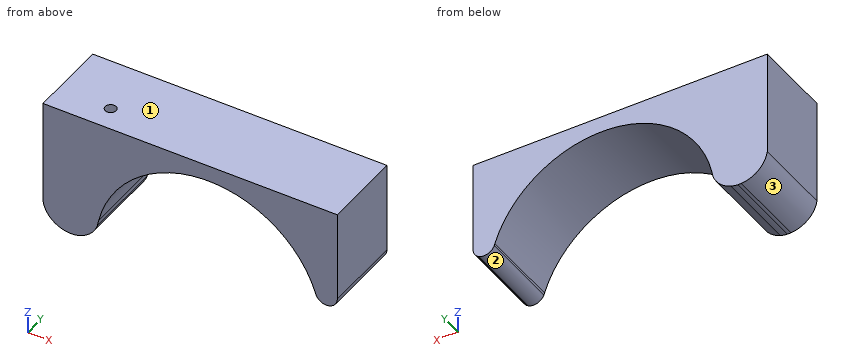
from build123d import *

# Parameters (mm, degrees)
F1_DEPTH = 15.875
F2_R     = 1.0922
F3_DEPTH = 12.7


# Not quite as in the source:
# - ends of sketch curves that miss each other by under 0.0002 mm in the source are joined


with BuildPart() as f1:
    # F0 (on Front) → F1 (new body)
    with BuildSketch(Plane.XZ):
        with BuildLine():
            ThreePointArc((21.0836389118, 7.0307037512), (21.1482213946, 6.8339854292), (21.2109684651, 6.6366739991))
            ThreePointArc((21.2109684651, 6.6366739991), (22.5210215532, 5.4318172042), (24.2927235367, 5.6020848515))
            Line((24.2927235367, 5.6020848515), (24.5564028335, 5.7779212439))
            ThreePointArc((24.5564028335, 5.7779212439), (24.6317726398, 5.83924537), (24.7043401509, 5.9038612541))
            ThreePointArc((24.7043401509, 5.9038612541), (24.1693958795, 7.8102690619), (23.4875772319, 9.6692148479))
            ThreePointArc((23.4875772319, 9.6692148479), (21.6017035502, 8.9730623402), (21.0836389118, 7.0307037512))
        make_face()
        with BuildLine():
            ThreePointArc((-25.3984668781, 0.2790703183), (-23.2092642977, 1.6544209311), (-21.8846396204, 3.8746836882))
            ThreePointArc((-21.8846396204, 3.8746836882), (-21.7800085202, 4.4251388519), (-21.6615343316, 4.9727814551))
            ThreePointArc((-21.6615343316, 4.9727814551), (-21.6412555699, 5.2455472098), (-21.6344904646, 5.5189820621))
            ThreePointArc((-21.6344904646, 5.5189820621), (-22.1206425964, 7.786095443), (-23.4936109358, 9.6545453128))
            ThreePointArc((-23.4936109358, 9.6545453128), (-24.8914383088, 5.057301545), (-25.3984668781, 0.2790703183))
        make_face()
        with BuildLine():
            Line((0, 25.4), (0, 22.225))
            ThreePointArc((0, 22.225), (12.9940993172, 18.0306408077), (21.0836389118, 7.0307037512))
            ThreePointArc((21.0836389118, 7.0307037512), (21.6017035502, 8.9730623402), (23.4875772319, 9.6692148479))
            ThreePointArc((23.4875772319, 9.6692148479), (14.1343896731, 21.1040050362), (0, 25.4))
        make_face()
        with BuildLine():
            ThreePointArc((-21.6615343316, 4.9727814551), (-13.8461286495, 17.3849172106), (0, 22.225))
            Line((0, 22.225), (0, 25.4))
            ThreePointArc((0, 25.4), (-14.1409785562, 21.099590647), (-23.4936109358, 9.6545453128))
            ThreePointArc((-23.4936109358, 9.6545453128), (-22.1206425964, 7.786095443), (-21.6344904646, 5.5189820621))
            ThreePointArc((-21.6344904646, 5.5189820621), (-21.6412555699, 5.2455472098), (-21.6615343316, 4.9727814551))
        make_face()
        with BuildLine():
            ThreePointArc((-26.8263954087, 0), (-26.1032119587, 0.0923630453), (-25.3984668781, 0.2790703183))
            ThreePointArc((-25.3984668781, 0.2790703183), (-24.8914383088, 5.057301545), (-23.4936109358, 9.6545453128))
            ThreePointArc((-23.4936109358, 9.6545453128), (-29.0403261825, 10.7200919312), (-32.6289507574, 6.3585310541))
            Line((-32.6289507574, 6.3585310541), (-32.6289507574, 4.6794330701))
            ThreePointArc((-32.6289507574, 4.6794330701), (-30.8909302127, 1.4347070449), (-27.501154691, 0))
            Line((-27.501154691, 0), (-26.8263954087, 0))
        make_face()
        with BuildLine():
            ThreePointArc((23.4875772319, 9.6692148479), (24.1693958795, 7.8102690619), (24.7043401509, 5.9038612541))
            ThreePointArc((24.7043401509, 5.9038612541), (25.2185681707, 6.630615454), (25.4000290489, 7.5022082908))
            ThreePointArc((25.4000290489, 7.5022082908), (24.8535428533, 8.9473198237), (23.4875772319, 9.6692148479))
        make_face()
        with BuildLine():
            ThreePointArc((23.4875772319, 9.6692148479), (24.8535428533, 8.9473198237), (25.4000290489, 7.5022082908))
            Line((25.4000290489, 7.5022082908), (25.4, 25.4))
            Line((25.4, 25.4), (0, 25.4))
            ThreePointArc((0, 25.4), (14.1343896731, 21.1040050362), (23.4875772319, 9.6692148479))
        make_face()
        with BuildLine():
            ThreePointArc((-23.4936109358, 9.6545453128), (-14.1409785562, 21.099590647), (0, 25.4))
            Line((0, 25.4), (-25.3993433231, 25.4))
            Line((-25.3993433231, 25.4), (-32.6289507574, 25.4))
            Line((-32.6289507574, 25.4), (-32.6289507574, 6.3585310541))
            ThreePointArc((-32.6289507574, 6.3585310541), (-29.0403261825, 10.7200919312), (-23.4936109358, 9.6545453128))
        make_face()
    extrude(amount=F1_DEPTH)

    # F2 (on face) → F3 (cut)
    with BuildSketch(Plane.XY.offset(25.4)):
        with Locations((-22.225, -11.1125)):
            Circle(F2_R)
    extrude(amount=-F3_DEPTH, mode=Mode.SUBTRACT)


solid = f1.part
Verification items for the finished model (mm, model axes). Face numbers are marked on the shaded views. Coordinates: 2 decimals unless noted, no trailing zeros. Write each loop counter-clockwise with the first axis right and the second up, starting at its lowest first coordinate (ties: lowest second). Pieces come first, ordered by that corner, then holes. Notation, with made-up numbers: M 16,-2 L 33,-2 A21 ccw 33,27 Z; hole C 66.5,26 d7. An arc over 180 degrees is marked long. Use CSV: the item, a comma, the result in double quotes.
Q1. Section check D-D, the plane x = 2. Enter the section's corners in (y, z) (3 decimals).
Computed values:
outline,"M -15.875,22.135 L 0,22.135 L 0,25.4 L -15.875,25.4 Z"
Q2. Thickness scan on line 1 along X through (y, z) = (-3.25, 7); line 2 along X through (y, z) = (-9.5, 7.25); line 3 along Z through (x, y) = (7, -1.5). Record the ranges inside material, lowest first. Write a range as [from, to].
Computed values:
line 1,"[-32.63, -21.09], [21.09, 25.34]"
line 2,"[-32.63, -21.01], [21.01, 25.39]"
line 3,"[21.09, 25.4]"
Q3. Go/stop test with flat-tipped pins: P1, Ø6, axis at x = 13, y = -2, coming from the -Z side; P2, Ø2.5, axis at x = -22.22, y = -11.11, coming from the -Z side; P3, Ø0.7, axis at x = -21.5, y = -11.5, coming from the +Z side; P4, Ø8, axis at x = -8.5, y = -13.5, coming from the -Z side. Record where each tip stops, or that it passes through.
Computed values:
P1,"z = 15.43"
P2,"z = 1.4"
P3,"z = 25.4"
P4,"z = 18.38"
Q4. Section check C-C, the plane z = 11.5. Enter the section's corners in (x, y) (3 decimals), and give its area (3 significant figures).
Computed values:
outline,"M -32.629,-15.875 L -19.018,-15.875 L -19.018,0 L -32.629,0 Z; M 19.018,-15.875 L 25.4,-15.875 L 25.4,0 L 19.018,0 Z"
area,"317 mm²"
Q5. Section check A-A, the plane z = 19. Enter the section's corners in (x, y) (1 decimal).
Computed values:
outline,"M -32.6,-15.9 L -11.5,-15.9 L -11.5,0 L -32.6,0 Z; M 11.5,-15.9 L 25.4,-15.9 L 25.4,0 L 11.5,0 Z; hole C -22.2,-11.1 d2.2"
Q6. Mould release check, pull along X, two halves, no side actions. Record for the marked faces 1, 2 and 3: pulls with the +X half, pulls with the -X half, needs draft (parallel to the pull), parting line crosses it, or undercut.
Computed values:
face 1,"needs draft"
face 2,"undercut"
face 3,"pulls with the -X half"
Q7. Section check B-B, the plane y = -5. Enter the section's corners in (x, z) (3 decimals).
Computed values:
outline,"M -32.629,4.679 A5.529 ccw -27.501,0 L -26.826,0 A5.529 ccw -21.885,3.875 A22.225 cw 21.084,7.031 A22.225 cw 21.211,6.637 A2.184 ccw 24.293,5.602 L 24.556,5.778 A2.184 ccw 25.4,7.502 L 25.4,25.4 L -32.629,25.4 Z"
